```python
from build123d import *

# Parameters (mm, degrees)
F3_DEPTH = 4.7625


# Not quite as in the source:
# - a length typed as a fraction of an inch, garbled in the dataset ("3 / 203.2 mm" for 3/8 in), is restored


with BuildPart() as f1:
    # F0 (on Front) → F1 (revolve)
    with BuildSketch(Plane.XZ):
        with BuildLine():
            Line((0, 76.2), (0, 0))
            Line((0, 0), (0, -4.7625))
            Line((0, -4.7625), (6.655733594, -4.7625))
            ThreePointArc((6.655733594, -4.7625), (8.2446462119, -3.314423226), (9.525, -1.5875))
            Line((9.525, -1.5875), (9.525, 0))
            Line((9.525, 0), (4.7244, 0))
            Line((4.7244, 0), (4.7244, 76.2))
            Line((4.7244, 76.2), (0, 76.2))
        make_face()
    revolve(axis=Axis((0, 0, 38.1), (0, 0, 1)))

    # F2 (on face) → F3 (cut)
    with BuildSketch(Plane(origin=(0, 0, -4.7625), x_dir=(1, 0, 0), z_dir=(0, 0, -1))):
        with BuildLine():
            Line((0, 7.9375), (5.2651418547, 7.9375))
            ThreePointArc((5.2651418547, 7.9375), (0, 9.525), (-5.2651418547, 7.9375))
            Line((-5.2651418547, 7.9375), (0, 7.9375))
        make_face()
    extrude(amount=-F3_DEPTH, mode=Mode.SUBTRACT)


solid = f1.part
```
Model file for the job. Use its own axes, mm. A direction names the side the tool comes from. Coordinates: 2 decimals unless noted, no trailing zeros. Loops run counter-clockwise (first coordinate to the right, second up) from the corner with the lowest first, then second, coordinate; pieces in that order, holes last. Notation, with made-up numbers: (87, 29) - (127, 29) arc R22 cw to (127, 36) - close; hole circle Ø5 at (59, 33). An arc over 180 degrees is marked (long way). Answer as a JSON object with one key per item and string values. Group by question number.
(1) Cut at B-B (x = 0). Give the cut face in (y, z) (1 decimal).
(2) Cut at C-C (z = 57). Give the cut face in (x, y).
(3) Probe line 1 along Z through (x, y) = (-4, -5); line 2 along X through (y, z) = (-3, 56); line 3 along Z through (x, y) = (7, 5.5). List the from-to ranges inside material, lowest first.
(4) Cut at A-A (y = 0). Give the cut face in (x, z) (1 decimal), then the cut area to 3 significant figures.
(5) Flat gauge pins, fed straight in: pin 1 (3 mm diameter, centred on x = -3.5, z = 34, fed in from +Y); pin 2 (8 mm diameter, centred on y = 4.5, z = 67, fed in from +X); pin 3 (1 mm diameter, centred on x = -6, y = 4.5, fed in from +Z). Where does each tip first touch, or does it go through?
(6) Tool access for faces 1 (the face through (0, -7.938, -1)), 2 (the face through (0, 5, 0)): list every direction of +Z, -Z, +X, -X, +Y, -Y with a clear straight run to the whole face (end or side of a thin tool).
Geometry says:
{
 "1": {"outline": "(-7.9, -3.6) arc R11.1 ccw to (-6.7, -4.8) - (6.7, -4.8) arc R11.1 ccw to (9.5, -1.6) - (9.5, 0) - (4.7, 0) - (4.7, 76.2) - (-4.7, 76.2) - (-4.7, 0) - (-7.9, 0) - close"},
 "2": {"outline": "circle Ø9.45 at (0, 0)"},
 "3": {"line 1": "z = -4.76 to 0", "line 2": "x = -3.65 to 3.65", "line 3": "z = -2.51 to 0"},
 "4": {"outline": "(-9.5, -1.6) arc R11.1 ccw to (-6.7, -4.8) - (6.7, -4.8) arc R11.1 ccw to (9.5, -1.6) - (9.5, 0) - (4.7, 0) - (4.7, 76.2) - (-4.7, 76.2) - (-4.7, 0) - (-9.5, 0) - close", "area": "803 mm^2"},
 "5": {"pin 1": "stops at y = 4.28", "pin 2": "stops at x = 4.7", "pin 3": "stops at z = 0"},
 "6": {"face 1": "+Z, -Z, +X, -X, -Y", "face 2": "+Z"}
}
